Can you work these out from the model? Positions are in its coordinate system, mm. Round coordinates to 2 decimals unless told otherwise and drop trailing zeros. Loops run counter-clockwise (first coordinate to the right, second up) from the corner with the lowest first, then second, coordinate; pieces in that order, holes last. Notation, with made-up numbers: (-33.5, 47.25) - (24.5, 47.25) arc R18 cw to (24.5, 65.25) - close; hole circle Ø7 at (38.25, -5.5). An arc over 180 degrees is marked (long way). Answer as CSV lines item,"result".
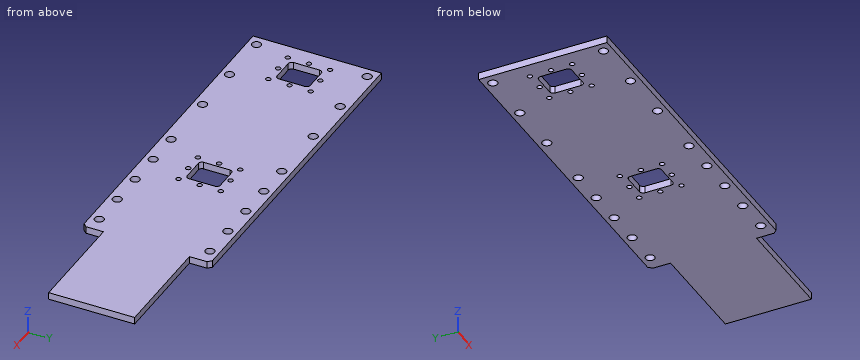
```python
from build123d import *

# Parameters (mm, degrees)
SKETCH_1_W          = 1255
SKETCH_1_H          = 364
EXTRUDE_1_DEPTH     = 20
SKETCH_2_W          = 305
SKETCH_2_H          = 60
CUT_EXTRUDE_1_DEPTH = 654.666772905
CHAMFER_1_SIZE      = 10
SKETCH_3_R          = 13
SKETCH_3_R_2        = 7
CUT_EXTRUDE_2_DEPTH = 20


with BuildPart() as part:
    # 草图1 → 凸台-拉伸1 (new body)
    with BuildSketch(Plane.XY):
        Rectangle(SKETCH_1_W, SKETCH_1_H)
    extrude(amount=-EXTRUDE_1_DEPTH)

    # 草图2 → 切除-拉伸1 (cut, through all)
    with BuildSketch(Plane.XY):
        with Locations((475, 152)):
            Rectangle(SKETCH_2_W, SKETCH_2_H)
        with Locations((475, -152)):
            Rectangle(SKETCH_2_W, SKETCH_2_H)
    extrude(amount=-CUT_EXTRUDE_1_DEPTH, mode=Mode.SUBTRACT)

    # 倒角1
    chamfer_1_edges = [part.edges().sort_by_distance(p)[0] for p in [
        (322.5, 182, -10),
        (322.5, -182, -10),
    ]]
    chamfer(chamfer_1_edges, length=CHAMFER_1_SIZE)

    # 草图3 → 切除-拉伸2 (cut)
    with BuildSketch(Plane.XY):
        with Locations((-597.5, 157)):
            Circle(SKETCH_3_R)
        with Locations((-447.5, 157)):
            Circle(SKETCH_3_R)
        with Locations((-297.5, 157)):
            Circle(SKETCH_3_R)
        with Locations((-122.5, 157)):
            Circle(SKETCH_3_R)
        with Locations((-22.5, 157)):
            Circle(SKETCH_3_R)
        with Locations((77.5, 157)):
            Circle(SKETCH_3_R)
        with Locations((177.5, 157)):
            Circle(SKETCH_3_R)
        with Locations((277.5, 157)):
            Circle(SKETCH_3_R)
        with Locations((277.5, -157)):
            Circle(SKETCH_3_R)
        with Locations((177.5, -157)):
            Circle(SKETCH_3_R)
        with Locations((77.5, -157)):
            Circle(SKETCH_3_R)
        with Locations((-22.5, -157)):
            Circle(SKETCH_3_R)
        with Locations((-122.5, -157)):
            Circle(SKETCH_3_R)
        with Locations((-297.5, -157)):
            Circle(SKETCH_3_R)
        with Locations((-447.5, -157)):
            Circle(SKETCH_3_R)
        with Locations((-597.5, -157)):
            Circle(SKETCH_3_R)
        with Locations((-581.5, 60)):
            Circle(SKETCH_3_R_2)
        with Locations((-527.5, 60)):
            Circle(SKETCH_3_R_2)
        with Locations((-473.5, 60)):
            Circle(SKETCH_3_R_2)
        with Locations((-473.5, 0)):
            Circle(SKETCH_3_R_2)
        with Locations((-581.5, 0)):
            Circle(SKETCH_3_R_2)
        with Locations((-581.5, -60)):
            Circle(SKETCH_3_R_2)
        with Locations((-527.5, -60)):
            Circle(SKETCH_3_R_2)
        with Locations((-473.5, -60)):
            Circle(SKETCH_3_R_2)
        with Locations((-81.5, 60)):
            Circle(SKETCH_3_R_2)
        with Locations((-27.5, 60)):
            Circle(SKETCH_3_R_2)
        with Locations((26.5, 60)):
            Circle(SKETCH_3_R_2)
        with Locations((26.5, 0)):
            Circle(SKETCH_3_R_2)
        with Locations((-81.5, 0)):
            Circle(SKETCH_3_R_2)
        with Locations((-81.5, -60)):
            Circle(SKETCH_3_R_2)
        with Locations((-27.5, -60)):
            Circle(SKETCH_3_R_2)
        with Locations((26.5, -60)):
            Circle(SKETCH_3_R_2)
        with BuildLine():
            Line((-58.5, 47), (3.5, 47))
            ThreePointArc((3.5, 47), (10.571067812, 44.071067812), (13.5, 37))
            Line((13.5, 37), (13.5, -37))
            ThreePointArc((13.5, -37), (10.571067812, -44.071067812), (3.5, -47))
            Line((3.5, -47), (-58.5, -47))
            ThreePointArc((-58.5, -47), (-65.571067812, -44.071067812), (-68.5, -37))
            Line((-68.5, -37), (-68.5, 37))
            ThreePointArc((-68.5, 37), (-65.571067812, 44.071067812), (-58.5, 47))
        make_face()
        with BuildLine():
            Line((-558.5, 47), (-496.5, 47))
            ThreePointArc((-496.5, 47), (-489.428932188, 44.071067812), (-486.5, 37))
            Line((-486.5, 37), (-486.5, -37))
            ThreePointArc((-486.5, -37), (-489.428932188, -44.071067812), (-496.5, -47))
            Line((-496.5, -47), (-558.5, -47))
            ThreePointArc((-558.5, -47), (-565.571067812, -44.071067812), (-568.5, -37))
            Line((-568.5, -37), (-568.5, 37))
            ThreePointArc((-568.5, 37), (-565.571067812, 44.071067812), (-558.5, 47))
        make_face()
    extrude(amount=-CUT_EXTRUDE_2_DEPTH, mode=Mode.SUBTRACT)


solid = part.part
```
Q1. I'm going to push flat-ended pins straight in: pin 1 Ø15.5 at (x, y) = (77.5, 157) entering from +Z; pin 2 Ø5 at (x, z) = (388.5, -18) entering from -Y. Where does each tip first touch, or does it pass through?
Checks:
pin 1,"through"
pin 2,"y = -122"
Q2. Imagine slicing it at C-C (y = 157). Count the separate pieces of the cut face and the enclosed holes in it, then the cut area to 3 significant figures.
Checks:
separate pieces,"9"
enclosed holes,"0"
area,"14,800 mm²"
Q3. If I drill on line 1 along Y through (x, z) = (-473.5, -16); line 2 along Y through (x, z) = (-297.5, -11.75); line 3 along X through (y, z) = (-28.5, -10.5), over which ranges is the centre line in solid material (lowest first)? Write a range as [from, to].
Checks:
line 1,"[-182, -67], [-53, -7], [7, 53], [67, 182]"
line 2,"[-182, -170], [-144, 144], [170, 182]"
line 3,"[-627.5, -568.5], [-486.5, -68.5], [13.5, 627.5]"
Q4. Imagine slicing it at B-B (x = 277.5). Write out the boundary of the cut face in (y, z), then the cut area to 3 significant figures.
Checks:
outline,"(-182, -20) - (-170, -20) - (-170, 0) - (-182, 0) - close; (-144, -20) - (144, -20) - (144, 0) - (-144, 0) - close; (170, -20) - (182, -20) - (182, 0) - (170, 0) - close"
area,"6,240 mm²"
Q5. Imagine slicing it at A-A (y = -26.5). Write out the boundary of the cut face in (x, z), then the cut area to 3 significant figures.
Checks:
outline,"(-627.5, -20) - (-568.5, -20) - (-568.5, 0) - (-627.5, 0) - close; (-486.5, -20) - (-68.5, -20) - (-68.5, 0) - (-486.5, 0) - close; (13.5, -20) - (627.5, -20) - (627.5, 0) - (13.5, 0) - close"
area,"21,800 mm²"
